Can you work these out from the drawing? Everything is in mm from the part's minimum corner. Give positions to 0.01 mm unless a question says otherwise; leave off trailing zeros. Write each loop counter-clockwise with the first axis right and the second up, starting at its lowest first coordinate (ties: lowest second). Pieces come first, ordered by that corner, then holes. Notation, with made-up numbers: (86, 77) - (138, 77) arc R20 cw to (138, 89) - close; hole circle Ø10 at (-10.75, -16.75). An arc over 180 degrees is marked (long way). Use a Markdown table: item, result.
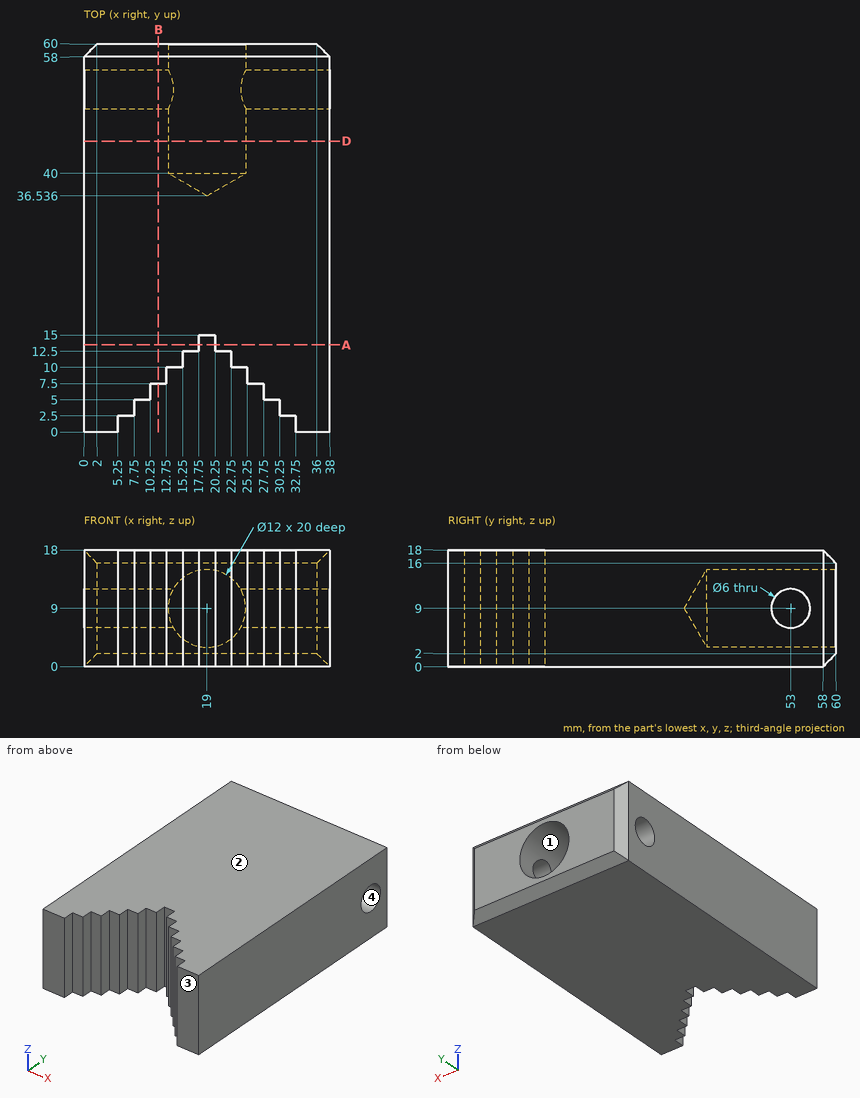
Item 1: If we section it at D-D, the plane y = 45: Write out the boundary of the cut face in (x, z).
Values:
| item | result |
|---|---|
| outline | (0, 0) - (38, 0) - (38, 18) - (0, 18) - close; hole circle Ø12 at (19, 9) |
Item 2: Will these pins go through, and if not, where does the flat tip stop? pin 1 Ø0.8 at (x, z) = (28.5, 8.5) entering from -Y; pin 2 Ø1.2 at (x, z) = (24.5, 9.5) entering from -Y; pin 3 Ø5.5 at (y, z) = (53, 9) entering from -X; pin 4 Ø3 at (x, z) = (13.5, 8) entering from -Y.
Values:
| item | result |
|---|---|
| pin 1 | stops at y = 5 |
| pin 2 | stops at y = 10 |
| pin 3 | passes through |
| pin 4 | stops at y = 7.5 |
Item 3: If we section it at B-B, the plane x = 11.5: Write out the boundary of the cut face in (y, z), plus the area to 3 significant figures.
Values:
| item | result |
|---|---|
| outline | (7.5, 0) - (58, 0) - (60, 2) - (60, 16) - (58, 18) - (7.5, 18) - close; hole circle Ø6 at (53, 9) |
| area | 913 mm2 |
Item 4: If we section it at A-A, the plane y = 13.5: Write out the boundary of the cut face in (x, z), plus the area to 3 significant figures.
Values:
| item | result |
|---|---|
| outline | (0, 0) - (17.75, 0) - (17.75, 18) - (0, 18) - close; (20.25, 0) - (38, 0) - (38, 18) - (20.25, 18) - close |
| area | 639 mm2 |
Item 5: I need wall thicknesses on line 1 along Z through (x, y) = (27, 53); line 2 along X through (y, z) = (42, 6); line 3 along Z through (x, y) = (19, 47.5). Which ranges of each line are inside material? Lowest first, please. Write a range as [from, to].
Values:
| item | result |
|---|---|
| line 1 | z = [0, 6], [12, 18] |
| line 2 | x = [0, 13.8], [24.2, 38] |
| line 3 | z = [0, 3], [15, 18] |
Item 6: Thinking about a two-plate mould opening in Z: for the marked faces 1, 2, 3 and 4, which applies, +Z half, -Z half, draft (parallel to the pull), parting line (faces both ways), or undercut?
Values:
| item | result |
|---|---|
| face 1 | undercut |
| face 2 | +Z half |
| face 3 | draft |
| face 4 | undercut |
